Can you work these out from the model? Positions are in its coordinate system, mm. Face numbers are marked on the shaded views. A direction names the side the tool comes from. Coordinates: 2 decimals unless noted, no trailing zeros. Loops run counter-clockwise (first coordinate to the right, second up) from the corner with the lowest first, then second, coordinate; pieces in that order, holes last. Notation, with made-up numbers: M 79,60 L 93,60 A19 cw 93,64 Z; hole C 49,40 d1. An arc over 180 degrees is marked long. Answer as a JSON object with one key per item and string values. Group by question number.
Item 1: Suppose I cut it at A-A (y = 0.5). Write out the boundary of the cut face in (x, z).
Item 2: If I drill on line 1 (Z direction, x = 0, y = -0.5); line 2 (Y direction, x = 4.5, z = 0.25); line 3 (X direction, y = 4, z = 5.5), over which ranges is the centre line in solid material (lowest first)?
Item 3: Which directions (+Z, -Z, +X, -X, +Y, -Y) give clear straight access to the entire face, cutting with the end or side of a thin tool? Please do the marked faces 1 and 2.
Item 4: I'm going to push flat-ended pins straight in: pin 1 Ø2 at (x, z) = (2, 5) entering from -Y; pin 2 Ø4 at (x, y) = (2, -16) entering from -Z. Where does each tip first touch, or does it pass through?
```python
from build123d import *

# Parameters (mm, degrees)
BOSS_EXTRUDE1_DEPTH = 5.5
SKETCH2_R           = 4
BOSS_EXTRUDE2_DEPTH = 30
FILLET1_R           = 0.4
CHAMFER1_SIZE       = 0.4


with BuildPart() as part:
    # Sketch1 → Boss-Extrude1 (new body)
    with BuildSketch(Plane(origin=(0, 0, 0), x_dir=(1, 0, 0), z_dir=(0, 1, 0))):
        Polygon((-3.75277675, -6.5), (3.75277675, -6.5), (7.505553499, 0), (3.75277675, 6.5), (-3.75277675, 6.5), (-7.505553499, 0), align=None)
    extrude(amount=BOSS_EXTRUDE1_DEPTH)

    # Sketch2 → Boss-Extrude2 (add)
    with BuildSketch(Plane.XZ):
        Circle(SKETCH2_R)
    extrude(amount=BOSS_EXTRUDE2_DEPTH)

    # Fillet1
    fillet1_edges = [part.edges().sort_by_distance(p)[0] for p in [
        (-4, 0, 0),
    ]]
    fillet(fillet1_edges, radius=FILLET1_R)

    # Chamfer1
    chamfer1_edges = [part.edges().sort_by_distance(p)[0] for p in [
        (-4, -30, 0),
    ]]
    chamfer(chamfer1_edges, length=CHAMFER1_SIZE)

    # Sketch3 → Cut-Revolve1 (revolve, cut)
    with BuildSketch(Plane(origin=(0, 0, 0), x_dir=(0, 0, -1), z_dir=(1, 0, 0))):
        Polygon((6.5, 5.5), (16.319077894, -0.169047265), (16.319077894, 5.5), align=None)
    revolve(axis=Axis((0, 0, 0), (0, 1, 0)), mode=Mode.SUBTRACT)


solid = part.part
```
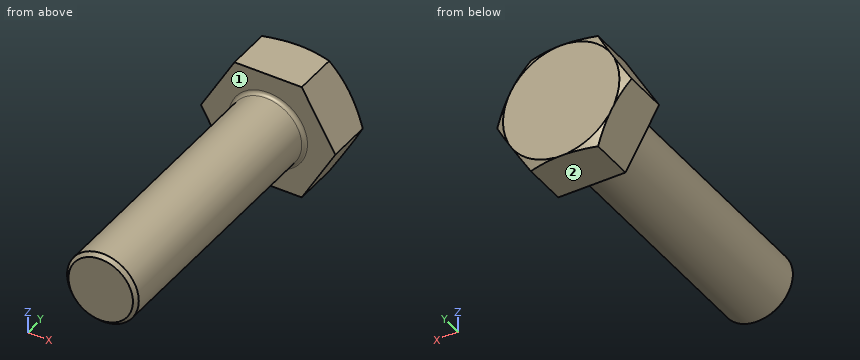
From the geometry:
{
 "1": {"outline": "M -7.51,0 L -3.75,-6.5 L 3.75,-6.5 L 7.51,0 L 3.75,6.5 L -3.75,6.5 Z"},
 "2": {"line 1": "-4 to 4", "line 2": "0 to 5.5", "line 3": "-4.33 to 4.33"},
 "3": {"face 1": "-Y", "face 2": "-Z, +X, -X, +Y, -Y"},
 "4": {"pin 1": "y = 0", "pin 2": "z = -4"}
}
